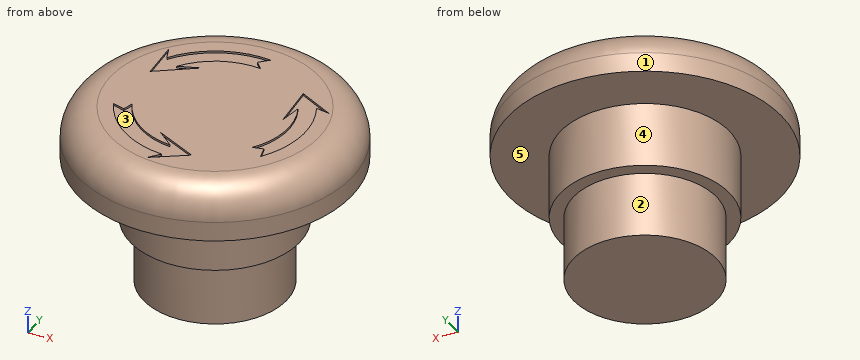
```python
from build123d import *

# Parameters (mm, degrees)
SKETCH_1_R               = 11
EXTRUDE_1_DEPTH          = 10
SKETCH_2_R               = 13
EXTRUDE_2_DEPTH          = 10
SKETCH_6_R               = 21
EXTRUDE_5_DEPTH          = 8
FILLET_4_R               = 5
CUT_EXTRUDE_3_DEPTH      = 0.3
PATTERN_CIRCULAR_1_COUNT = 3


with BuildPart() as part:
    # Sketch 1 → Extrude 1 (new body)
    with BuildSketch(Plane.XY):
        Circle(SKETCH_1_R)
    extrude(amount=EXTRUDE_1_DEPTH)

    # Sketch 2 → Extrude 2 (add)
    with BuildSketch(Plane.XY.offset(10)):
        Circle(SKETCH_2_R)
    extrude(amount=EXTRUDE_2_DEPTH)

    # Sketch 6 → Extrude 5 (add)
    with BuildSketch(Plane.XY.offset(20)):
        Circle(SKETCH_6_R)
    extrude(amount=EXTRUDE_5_DEPTH)

    # Fillet 4
    fillet_4_edges = [part.edges().sort_by_distance(p)[0] for p in [
        (-21, 0, 28),
    ]]
    fillet(fillet_4_edges, radius=FILLET_4_R)

    # Sketch 7 → Cut-Extrude 3 (cut)
    with BuildSketch(Plane.XY.offset(28)):
        with BuildLine():
            Line((-9.304992191, 6.340429284), (-6.090228266, 7.590754313))
            Line((-6.090228266, 7.590754313), (-11.877072904, 3.512738797))
            Line((-11.877072904, 3.512738797), (-12.271255314, 9.560904356))
            Line((-12.271255314, 9.560904356), (-11.499666165, 7.577038638))
            ThreePointArc((-11.499666165, 7.577038638), (-5.993368065, 12.398926391), (1.205826183, 13.718593938))
            Line((1.205826183, 13.718593938), (-0.151715423, 12.361052332))
            Line((-0.151715423, 12.361052332), (0.993407881, 11.215929028))
            ThreePointArc((0.993407881, 11.215929028), (-4.818011299, 10.176968621), (-9.304992191, 6.340429284))
        make_face()
    cut_extrude_3 = extrude(amount=-CUT_EXTRUDE_3_DEPTH, mode=Mode.SUBTRACT)

    # Pattern Circular 1: Cut-Extrude 3 ×3 about axis
    pattern_circular_1_axis = Axis((0, 0, 0), (0, 0, 1))
    for i in range(1, PATTERN_CIRCULAR_1_COUNT):
        add(cut_extrude_3.rotate(pattern_circular_1_axis, i * 360 / PATTERN_CIRCULAR_1_COUNT), mode=Mode.SUBTRACT)


solid = part.part
```
Verification items for the finished model (mm, model axes). Face numbers are marked on the shaded views. A direction names the side the tool comes from. Round coordinates to 2 decimals unless told otherwise and drop trailing zeros. Loops run counter-clockwise (first coordinate to the right, second up) from the corner with the lowest first, then second, coordinate; pieces in that order, holes last. Notation, with made-up numbers: (-29.5, 32) -> (-24.5, 32) arc R26 cw to (-24.5, 61) -> close; hole circle Ø6 at (73.25, 87.25). An arc over 180 degrees is marked (long way). Answer as a JSON object with one key per item and string values.
Q1. Section check C-C (z = 15). Record the boundary of the cut face in (x, y), then the cut area to 3 significant figures.
Data:
{"outline": "circle Ø26 at (0, 0)", "area": "531 mm2"}
Q2. Access from +Z, -Z, +X, -X, +Y, -Y to the whole of each face (thin tool, end or side, straight path). Record for the marked faces 1 and 2.
Data:
{"face 1": "+Z, -Z", "face 2": "-Z"}
Q3. Scan lines: line 1 (Z direction, x = -11.5, y = 11); line 2 (Z direction, x = -5, y = 17); line 3 (X direction, y = 10.5, z = 20.5). Record each from-to range of solid material in increasing order. Write a range as from..to.
Data:
{"line 1": "z = 20..28", "line 2": "z = 20..27.69", "line 3": "x = -18.19..18.19"}
Q4. Go/stop test with flat-tipped pins: P1, Ø10, axis at x = 14.5, z = 21, coming from the +Y side; P2, Ø3, axis at y = 15, z = 21, coming from the +X side; P3, Ø5, axis at x = -7.5, z = 10, coming from the -Y side. Record where each tip stops, or that it passes through.
Data:
{"P1": "stops at y = 18.73", "P2": "stops at x = 16.09", "P3": "stops at y = -12"}
Q5. Section check B-B (z = 2). Record the boundary of the cut face in (x, y).
Data:
{"outline": "circle Ø22 at (0, 0)"}
Q6. Draft check along X on the marked faces 3, 4 and 5. Enter one of: pulls with the +X half, pulls with the -X half, needs draft (parallel to the pull), parting line crosses it, or undercut.
Data:
{"face 3": "undercut", "face 4": "parting line crosses it", "face 5": "needs draft"}
Q7. Section check A-A (y = 0). Record the boundary of the cut face in (x, z).
Data:
{"outline": "(-21, 20) -> (-13, 20) -> (-13, 10) -> (-11, 10) -> (-11, 0) -> (11, 0) -> (11, 10) -> (13, 10) -> (13, 20) -> (21, 20) -> (21, 23) arc R5 ccw to (16, 28) -> (13.77, 28) -> (13.77, 27.7) -> (11.26, 27.7) -> (11.26, 28) -> (-16, 28) arc R5 ccw to (-21, 23) -> close"}
